Could you check a few things on this model? Use its own coordinates, in mm. A direction names the side the tool comes from. Give positions to 0.01 mm unless a question says otherwise; leave off trailing zeros. Loops run counter-clockwise (first coordinate to the right, second up) from the corner with the lowest first, then second, coordinate; pieces in that order, holes last. Notation, with made-up numbers: M 55,1.5 L 99,1.5 A13 ccw 99,15.5 Z; hole C 8.25,89.25 d6. An arc over 180 degrees is marked long. Write each question's results on one line, items separated by ' | '. Start each with the question number.
from build123d import *

# Parameters (mm, degrees)
CROQUIS1_W              = 9.4
CROQUIS1_H              = 16
SALIENTE_EXTRUIR1_DEPTH = 3
CROQUIS2_W              = 3.3
CROQUIS2_H              = 8.5
CORTAR_EXTRUIR1_DEPTH   = 3
SALIENTE_EXTRUIR2_DEPTH = 3
REDONDEO1_R             = 0.5


with BuildPart() as part:
    # Croquis1 → Saliente-Extruir1 (new body)
    with BuildSketch(Plane(origin=(0, 0, 0), x_dir=(0, 0, -1), z_dir=(1, 0, 0))):
        Rectangle(CROQUIS1_W, CROQUIS1_H)
    extrude(amount=SALIENTE_EXTRUIR1_DEPTH)

    # Croquis2 → Cortar-Extruir1 (cut)
    with BuildSketch(Plane(origin=(3, 0, 0), x_dir=(0, 0, -1), z_dir=(1, 0, 0))):
        with Locations((0, -3.75)):
            Rectangle(CROQUIS2_W, CROQUIS2_H)
    extrude(amount=-CORTAR_EXTRUIR1_DEPTH, mode=Mode.SUBTRACT)

    # Croquis4 → Saliente-Extruir2 (add)
    with BuildSketch(Plane(origin=(3, 0, 0), x_dir=(0, 0, -1), z_dir=(1, 0, 0))):
        Polygon((4.7, 4.391798286), (4.7, 1.391798286), (9.2, 1.391798286), (11.82874383, 4.204558046), (10.369105711, 6.327401467), (7.869105711, 6.327401467), (9.2, 4.391798286), align=None)
    extrude(amount=-SALIENTE_EXTRUIR2_DEPTH)

    # Redondeo1
    redondeo1_edges = [part.edges().sort_by_distance(p)[0] for p in [
        (1.5, -8, 1.65),
        (1.5, 0.5, 1.65),
        (1.5, 0.5, -1.65),
        (1.5, -8, -1.65),
        (1.5, 4.391798286, -4.7),
        (1.5, 4.391798286, -9.2),
        (1.5, 6.327401467, -7.869105711),
        (1.5, 6.327401467, -10.369105711),
        (1.5, 4.204558046, -11.82874383),
        (1.5, 1.391798286, -9.2),
        (1.5, 1.391798286, -4.7),
        (1.5, 8, 4.7),
        (1.5, 8, -4.7),
        (1.5, -8, -4.7),
        (1.5, -8, 4.7),
    ]]
    fillet(redondeo1_edges, radius=REDONDEO1_R)


solid = part.part
1) Thinking about a two-plate mould opening in Z: for faces 1 (the face through (1, -3, -4.7)), 2 (the face through (2, 0.5, 0)), 3 (the face through (1, -8, -3)), 4 (the face through (2, -4, -1.65)), which applies, pulls with the +Z half, pulls with the -Z half, needs draft (parallel to the pull), parting line crosses it, or undercut?
2) Please list where these lines run through material, in increasing order: line 1 (Z direction, x = 0.5, y = -6.75); line 2 (Y direction, x = 2.65, z = -8); line 3 (Y direction, x = 2.45, z = -4.25). Write a range as from..to.
3) If we section it at C-C on z = 0.75: Write out the boundary of the cut face in (x, y), plus the area to 3 significant figures.
4) Which directions (+Z, -Z, +X, -X, +Y, -Y) give clear straight access to the entire face, cutting with the end or side of a thin tool? Please do faces 5 (the face through (2, 6.327, -9)), 6 (the face through (2, 1.392, -7)), 7 (the face through (2, -4, 1.65)), 8 (the face through (1, 6, -4.7)).
5) I'm going to push flat-ended pins straight in: P1, Ø0.9, axis at x = 1, y = -2.5, coming from the -Z side; P2, Ø1.4, axis at x = 1.5, z = -9.5, coming from the +Y side; P3, Ø0.8, axis at x = 1.5, y = 5.5, coming from the -Z side. Where does each tip first touch, or does it pass through?
6) If we section it at D-D on y = 7: Write out the boundary of the cut face in (x, z).
7) If we section it at A-A on y = -3: Write out the boundary of the cut face in (x, z), plus the area to 3 significant figures.
Calculated:
1) face 1: pulls with the -Z half | face 2: undercut | face 3: needs draft | face 4: undercut
2) line 1: z = -4.7..-1.65, 1.65..4.7 | line 2: y = 1.39..4.39 | line 3: y = -8..8
3) outline: M 0,0.5 L 3,0.5 L 3,8 L 0,8 Z | area: 22.5 mm2
4) face 5: -Z, +X, -X, +Y | face 6: -Z, +X, -X, -Y | face 7: +X, -X, -Y | face 8: +X, -X, +Y
5) P1: stops at z = -4.7 | P2: stops at y = 6.33 | P3: stops at z = -11.21
6) outline: M 0,-4.7 L 3,-4.7 L 3,4.7 L 0,4.7 Z
7) outline: M 0,-4.7 L 3,-4.7 L 3,-1.65 L 0,-1.65 Z; M 0,1.65 L 3,1.65 L 3,4.7 L 0,4.7 Z | area: 18.3 mm2
